The model under review builds one solid part; all positions refer to its coordinate system, in mm. Face numbers are marked on the shaded views. Give positions to 0.01 mm unless a question says otherwise; leave off trailing zeros. Order: outer loops, then holes, each group sorted by start corner. A loop starts at its lowest first (then second) coordinate and runs counter-clockwise, first axis right, second up. Notation, with made-up numbers: (29.25, -26.75) - (35.25, -26.75) arc R23 ccw to (35.25, 6.25) - close; hole circle Ø9 at (58, 38.25). An arc over 180 degrees is marked (long way). Use CSV: the item, a comma, the result in double quotes. Start each with the question number.
1. To check wall thickness, follow line 1 (Y direction, x = 0, z = 2.5); line 2 (Y direction, x = 28.5, z = 0.7); line 3 (X direction, y = 8, z = 0.75). State the ranges of each line that lie inside material, in increasing order. Write a range as [from, to].
2. Take a section at B-B, the plane z = 5. State the section outline as (x, y) points, then the cut area to 3 significant figures.
3. Take a section at C-C, the plane y = 0. Count the separate pieces of the cut face and the enclosed holes in it, then the cut area to 3 significant figures.
4. For pin 1 (2 mm diameter, centred on x = 4, z = 4.5, fed in from +Y); pin 2 (1.5 mm diameter, centred on x = 12.5, z = 2, fed in from +Y); pin 3 (1.3 mm diameter, centred on x = 14.5, y = 25.5, fed in from -Z), all flat-tipped, find the tip position at first contact; note any pin that passes through.
5. Draft analysis for pull direction X (two halves, no side actions). For the marked faces 1, 2 and 3, state which applies: released by +X, released by -X, zero draft, split by the parting line, or undercut.
6. Take a section at A-A, the plane x = 0. State the section outline as (y, z) points.
```python
from build123d import *

# Parameters (mm, degrees)
SKETCH1_R                    = 33
MAIN_BODY_DEPTH              = 7
SKETCH2_R                    = 22
OPTICAL_CUTOUT_DEPTH         = 8
SKETCH3_R                    = 25.4
WINDOW_CUTOUT_DEPTH          = 5
SKETCH4_R                    = 1.2
CUT_EXTRUDE3_DEPTH           = 8
SKETCH5_R                    = 2.1
CUT_EXTRUDE4_DEPTH           = 2
CIRCULAR_PATTERN_COUNT       = 6
BUBBLE_CONTROL_CHAMFER_SIZE  = 1
BUBBLE_CONTROL_CHAMFER_SIZE2 = 2
CHAMFER1_SIZE                = 0.3


with BuildPart() as part:
    # Sketch1 → Main Body (new body)
    with BuildSketch(Plane.XY):
        Circle(SKETCH1_R)
    extrude(amount=MAIN_BODY_DEPTH)

    # Sketch2 → Optical Cutout (cut, through all)
    with BuildSketch(Plane.XY.offset(7)):
        Circle(SKETCH2_R)
    extrude(amount=-OPTICAL_CUTOUT_DEPTH, mode=Mode.SUBTRACT)

    # Sketch3 → Window Cutout (cut)
    with BuildSketch(Plane.XY.offset(7)):
        Circle(SKETCH3_R)
    extrude(amount=-WINDOW_CUTOUT_DEPTH, mode=Mode.SUBTRACT)

    # Sketch4 → Cut-Extrude3 (cut, through all)
    with BuildSketch(Plane(origin=(0, 0, 0), x_dir=(-1, 0, 0), z_dir=(0, 0, -1))):
        with Locations((14.25, 24.681724008)):
            Circle(SKETCH4_R)
    cut_extrude3 = extrude(amount=-CUT_EXTRUDE3_DEPTH, mode=Mode.SUBTRACT)

    # Sketch5 → Cut-Extrude4 (cut)
    with BuildSketch(Plane(origin=(0, 0, 0), x_dir=(-1, 0, 0), z_dir=(0, 0, -1))):
        with Locations((14.25, 24.681724008)):
            Circle(SKETCH5_R)
    cut_extrude4 = extrude(amount=-CUT_EXTRUDE4_DEPTH, mode=Mode.SUBTRACT)

    # Circular Pattern: Cut-Extrude3, Cut-Extrude4 ×6 about axis
    circular_pattern_axis = Axis((0, 0, 0), (0, 0, 1))
    for i in range(1, CIRCULAR_PATTERN_COUNT):
        add(cut_extrude3.rotate(circular_pattern_axis, i * 360 / CIRCULAR_PATTERN_COUNT), mode=Mode.SUBTRACT)
        add(cut_extrude4.rotate(circular_pattern_axis, i * 360 / CIRCULAR_PATTERN_COUNT), mode=Mode.SUBTRACT)

    # Bubble Control Chamfer
    bubble_control_chamfer_edges = [part.edges().sort_by_distance(p)[0] for p in [
        (-22, 0, 0),
    ]]
    bubble_control_chamfer_side = [part.faces().sort_by_distance(p)[0] for p in [
        (-22, 0, 1),
    ]]
    chamfer(bubble_control_chamfer_edges, length=BUBBLE_CONTROL_CHAMFER_SIZE, length2=BUBBLE_CONTROL_CHAMFER_SIZE2, reference=bubble_control_chamfer_side[0])

    # Chamfer1
    chamfer1_edges = [part.edges().sort_by_distance(p)[0] for p in [
        (-25.4, 0, 7),
        (-22, 0, 2),
        (-33, 0, 0),
        (-33, 0, 7),
    ]]
    chamfer(chamfer1_edges, length=CHAMFER1_SIZE)


solid = part.part
```
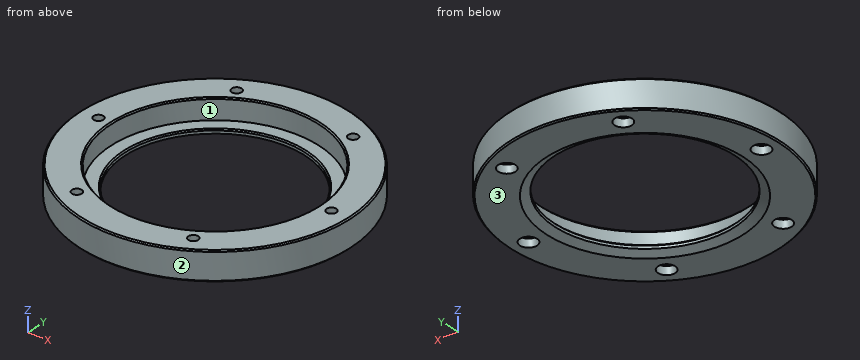
Determined:
1,line 1,"y = [-33, -25.4], [25.4, 33]"
1,line 2,"y = [-16.64, -2.1], [2.1, 16.64]"
1,line 3,"x = [-32.02, -21.03], [21.03, 32.02]"
2,outline,"circle Ø66 at (0, 0); hole circle Ø2.4 at (-28.5, 0); hole circle Ø50.8 at (0, 0); hole circle Ø2.4 at (-14.25, -24.68); hole circle Ø2.4 at (-14.25, 24.68); hole circle Ø2.4 at (14.25, -24.68); hole circle Ø2.4 at (14.25, 24.68); hole circle Ø2.4 at (28.5, 0)"
2,area,"1,370 mm²"
3,separate pieces,"4"
3,enclosed holes,"0"
3,area,"76.8 mm²"
4,pin 1,"stops at y = 32.86"
4,pin 2,"stops at y = 30.84"
4,pin 3,"stops at z = 2"
5,face 1,"undercut"
5,face 2,"split by the parting line"
5,face 3,"zero draft"
6,outline,"(-33, 0.3) - (-32.7, 0) - (-24, 0) - (-22, 1) - (-22, 1.7) - (-22.3, 2) - (-25.4, 2) - (-25.4, 6.7) - (-25.7, 7) - (-32.7, 7) - (-33, 6.7) - close; (22, 1) - (24, 0) - (32.7, 0) - (33, 0.3) - (33, 6.7) - (32.7, 7) - (25.7, 7) - (25.4, 6.7) - (25.4, 2) - (22.3, 2) - (22, 1.7) - close"
